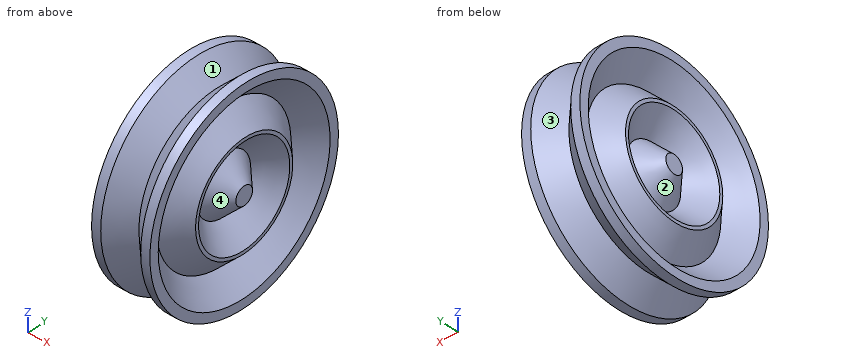
```python
from build123d import *


with BuildPart() as f1:
    # F0 (on Top) → F1 (revolve)
    with BuildSketch(Plane.XY):
        Polygon((2.828427, 0), (0, 0), (0, -2.828427), (6.335786, -9.164214), (0, -15.5), (0, -16.5), (6.335786, -22.835786), (0, -29.171573), (0, -32), (2.828427, -32), (9, -25.828427), (15.171573, -32), (18, -32), (18, -29.171573), (11.664214, -22.835786), (18, -16.5), (18, -15.5), (11.664214, -9.164214), (18, -2.828427), (18, 0), (15.171573, 0), (9, -6.171573), align=None)
        Polygon((5.156854, -16), (9, -12.156854), (12.843146, -16), (9, -19.843146), align=None, mode=Mode.SUBTRACT)
        Polygon((12.843146, -16), (9, -12.156854), (5.156854, -16), (9, -19.843146), align=None)
    revolve(axis=Axis((16.585786, 0, 0), (1, 0, 0)))


solid = f1.part
```
Model file for the job. Use its own axes, mm. Face numbers are marked on the shaded views. A direction names the side the tool comes from. Round coordinates to 2 decimals unless told otherwise and drop trailing zeros. Write each loop counter-clockwise with the first axis right and the second up, starting at its lowest first coordinate (ties: lowest second). Pieces come first, ordered by that corner, then holes. Notation, with made-up numbers: (79.25, 9.5) -> (125.25, 9.5) arc R14 cw to (125.25, 31.5) -> close; hole circle Ø4 at (36.25, 51). An arc over 180 degrees is marked (long way). Answer as CSV lines item,"result".
1. Mould opens along Y. For the marked faces 1 and 2 say: +Y half, -Y half, draft (parallel to the pull), parting line (faces both ways), or undercut.
Resolved:
face 1,"parting line"
face 2,"undercut"
2. Slice it at A-A, the plane x = 12.75. List the corners of the cut face in (y, z), plus the area to 3 significant figures.
Resolved:
outline,"circle Ø59.16 at (0, 0); circle Ø43.5 at (0, 0); circle Ø16.16 at (0, 0); hole circle Ø47.84 at (0, 0); hole circle Ø20.5 at (0, 0); hole circle Ø4.84 at (0, 0)"
area,"2,290 mm²"
3. Drill centre lines: line 1 (Z direction, x = 15, y = 13.5); line 2 (Z direction, x = 2, y = 10); line 3 (Z direction, x = 2.75, y = 10.5). Where is each one in solid material? Low to high.
Resolved:
line 1,"-28.82 to -22.42, -14.07 to 14.07, 22.42 to 28.82"
line 2,"-30.4 to -25.26, -15.56 to -9.07, 9.07 to 15.56, 25.26 to 30.4"
line 3,"-30.23 to -24.25, -16.13 to -7.23, 7.23 to 16.13, 24.25 to 30.23"
4. Tool access for the marked faces 3 and 4: list every direction of +Z, -Z, +X, -X, +Y, -Y with a clear straight run to the whole face (end or side of a thin tool).
Resolved:
face 3,"none"
face 4,"+X"
5. Pin check, flat tips, straight feed: pin 1 Ø5 at (x, y) = (6.5, -21) entering from +Z; pin 2 Ø5 at (x, z) = (12, -0.5) entering from +Y; pin 3 Ø1.5 at (x, z) = (6.5, -15) entering from -Y. Stop position of each tip, or through.
Resolved:
pin 1,"z = 23.24"
pin 2,"y = 31.32"
pin 3,"y = -25.02"
6. Slice it at B-B, the plane x = 4.5. List the corners of the cut face in (y, z), plus the area to 3 significant figures.
Resolved:
outline,"circle Ø60.66 at (0, 0); circle Ø42 at (0, 0); circle Ø14.66 at (0, 0); hole circle Ø49.34 at (0, 0); hole circle Ø22 at (0, 0); hole circle Ø3.34 at (0, 0)"
area,"2,140 mm²"
